from build123d import *

# Parameters (mm, degrees)
SKETCH1_W           = 60.00000000000001
SKETCH1_H           = 32
BOSS_EXTRUDE1_DEPTH = 5.3
BOSS_EXTRUDE2_DEPTH = 60
SKETCH4_R           = 5.050000000000001
BOSS_EXTRUDE3_DEPTH = 5
BOSS_EXTRUDE4_DEPTH = 15
BOSS_EXTRUDE5_DEPTH = 5.3
CUT_EXTRUDE1_DEPTH  = 10
CUT_EXTRUDE2_DEPTH  = 5
CUT_EXTRUDE3_DEPTH  = 5
CUT_EXTRUDE4_START  = -15
SKETCH4_4_R         = 5.050000000000001
CUT_EXTRUDE4_DEPTH  = 15
FILLET1_R           = 1


with BuildPart() as part:
    # Sketch1 → Boss-Extrude1 (new body)
    with BuildSketch(Plane.XY):
        with Locations((30.000000000000004, 16)):
            Rectangle(SKETCH1_W, SKETCH1_H)
    extrude(amount=BOSS_EXTRUDE1_DEPTH)

    # Sketch3 → Boss-Extrude2 (add)
    with BuildSketch(Plane.ZY):
        Polygon((5.29999999999999, 32), (5.29999999999999, 32.5), (0, 32), align=None)
        Polygon((5.3, -0.5), (5.3, 0), (0, 0), align=None)
    extrude(amount=-BOSS_EXTRUDE2_DEPTH)

    # Sketch4 → Boss-Extrude3 (add)
    # profile 1 of 9: a face of its own
    with BuildSketch(Plane.XY.offset(5.3)):
        Polygon((1.3289678218773275, 32.5), (24.983548935155518, 32.5), (1.5086509412101563, 34.55378745189766), align=None)
    # profile 2 of 9: a face of its own
    with BuildSketch(Plane.XY.offset(5.3)):
        Polygon((0, 2.5635425050841554), (35.01645106484395, -0.4999999999999578), (58.671032178122694, -0.5000000000000004), (59.999999999999964, 14.690171712744215), (60, 29.43645749491585), (24.983548935155518, 32.5), (1.3289678218773275, 32.5), (-4e-15, 17.309828287255154), align=None)
        with Locations((30, 16)):
            Circle(SKETCH4_R, mode=Mode.SUBTRACT)
    # profile 3 of 9: a face of its own
    with BuildSketch(Plane.XY.offset(5.3)):
        Polygon((0, -0.5000000000000004), (35.01645106484395, -0.5000000000000004), (0, 2.5635425050841554), align=None)
    # profile 4 of 9: a face of its own
    with BuildSketch(Plane.XY.offset(5.3)):
        Polygon((58.055570345051585, -7.534760942356384), (58.49134905878986, -2.553787451897688), (35.01645106484395, -0.4999999999999578), (0, -0.5000000000000004), (0, 2.5635425050841576), (-1.2803328267148615, 2.675557112961807), (-1.7161115404531533, -2.3054163774969894), align=None)
    # profile 5 of 9: a face of its own
    with BuildSketch(Plane.XY.offset(5.3)):
        Polygon((35.01645106484395, -0.4999999999999578), (58.49134905878986, -2.5537874518976778), (58.671032178122694, -0.5000000000000071), align=None)
    # profile 6 of 9: a face of its own
    with BuildSketch(Plane.XY.offset(5.3)):
        Polygon((59.999999999999964, 14.690171712744215), (61.28033282671488, 29.324442887038195), (60, 29.436457494915846), align=None)
    # profile 7 of 9: a face of its own
    with BuildSketch(Plane.XY.offset(5.3)):
        Polygon((24.983548935155518, 32.5), (60, 29.436457494915846), (60, 32.5), align=None)
    # profile 8 of 9: a face of its own
    with BuildSketch(Plane.XY.offset(5.3)):
        Polygon((60, 29.436457494915846), (61.28033282671488, 29.324442887038195), (61.71611154045317, 34.305416377497), (1.944429654948438, 39.5347609423564), (1.5086509412101552, 34.55378745189767), (24.983548935155518, 32.5), (60, 32.5), align=None)
    # profile 9 of 9: a face of its own
    with BuildSketch(Plane.XY.offset(5.3)):
        Polygon((-1.2803328267148615, 2.675557112961807), (0, 2.5635425050841554), (0, 17.309828287255158), align=None)
    extrude(amount=BOSS_EXTRUDE3_DEPTH)

    # Sketch4<3> → Boss-Extrude4 (add)
    with BuildSketch(Plane.XY.offset(5.3)):
        Polygon((60, 29.436457494915846), (61.28033282671488, 29.324442887038195), (61.71611154045317, 34.305416377497), (1.944429654948438, 39.5347609423564), (1.5086509412101552, 34.55378745189767), (24.983548935155518, 32.5), (60, 32.5), align=None)
        Polygon((24.983548935155518, 32.5), (60, 29.436457494915846), (60, 32.5), align=None)
        Polygon((58.055570345051585, -7.534760942356384), (58.49134905878986, -2.553787451897688), (35.01645106484395, -0.4999999999999578), (0, -0.5000000000000004), (0, 2.5635425050841576), (-1.2803328267148615, 2.675557112961807), (-1.7161115404531533, -2.3054163774969894), align=None)
        Polygon((0, -0.5000000000000004), (35.01645106484395, -0.5000000000000004), (0, 2.5635425050841554), align=None)
    extrude(amount=BOSS_EXTRUDE4_DEPTH)

    # Sketch6 → Boss-Extrude5 (add)
    with BuildSketch(Plane(origin=(0, 0, 5.3), x_dir=(-1, 0, 0), z_dir=(0, 0, -1))):
        Polygon((-2.2e-16, 17.3098282872552), (0, -0.5000000000000004), (1.558158074478129, -0.499999999999997), align=None)
        Polygon((-60.00000000000001, 14.690171712744698), (-60, 32.5), (-61.55815807447815, 32.5), align=None)
    extrude(amount=BOSS_EXTRUDE5_DEPTH)

    # Sketch5 → Cut-Extrude1 (cut)
    with BuildSketch(Plane.XY.offset(5.3)):
        Polygon((58.671032178122694, -0.5000000000000004), (60, -0.5000000000000004), (60.00000000000001, 14.690171712744698), align=None)
        Polygon((1.328967821877318, 32.5), (0, 32.5), (2.2e-16, 17.3098282872552), align=None)
    extrude(amount=-CUT_EXTRUDE1_DEPTH, mode=Mode.SUBTRACT)

    # Sketch7 → Cut-Extrude2 (cut)
    with BuildSketch(Plane(origin=(0, 0, 0), x_dir=(0, 0, -1), z_dir=(1, -1e-17, 0))):
        Polygon((0, -0.5000000000000004), (3.2e-16, 3.5e-15), (-5.3, -0.5000000000000004), align=None)
    extrude(amount=-CUT_EXTRUDE2_DEPTH, mode=Mode.SUBTRACT)

    # Sketch8 → Cut-Extrude3 (cut)
    with BuildSketch(Plane.ZY.offset(-60.000000000000014)):
        Polygon((5.299999999999987, 32.49999999999998), (0, 31.99999999999998), (0, 32.49999999999998), align=None)
    extrude(amount=-CUT_EXTRUDE3_DEPTH, mode=Mode.SUBTRACT)

    # Sketch4<4> → Cut-Extrude4 (cut)
    with BuildSketch(Plane.XY.offset(5.3).offset(CUT_EXTRUDE4_START)):
        with Locations(Location((30, 16, 0), (0, 0, 180))):
            Circle(SKETCH4_4_R)
    extrude(amount=CUT_EXTRUDE4_DEPTH, mode=Mode.SUBTRACT)

    # Fillet1
    fillet1_edges = [part.edges().sort_by_distance(p)[0] for p in [
        (-1.637134807465641, -1.402708188748493, 5.3),
        (58.692904344004184, -0.25000000000000244, 2.65),
        (1.307095655995838, 32.25, 2.6499999999999977),
        (-0.11459512630040658, 16.000000000000004, 0),
        (-1.5362859085966487, -0.24999999999999853, 2.65),
        (60.11459512630042, 15.999999999999996, 0),
        (61.53628590859667, 32.25, 2.6499999999999937),
        (35.05, 16, 0),
        (58.36330126158714, -4.017380471178193, 5.3),
        (61.63713480746566, 33.4027081887485, 5.3),
        (31.830270597700803, 36.920088659926705, 5.3),
        (1.6366987384128773, 36.0173804711782, 5.299999999999997),
        (1.944429654948438, 39.5347609423564, 12.8),
        (28.169729402299218, -4.920088659926687, 5.3),
        (-1.7161115404531533, -2.3054163774969894, 12.8),
        (58.055570345051585, -7.534760942356385, 12.8),
        (61.71611154045317, 34.305416377497, 12.8),
        (24.95, 16, 10.3),
        (31.399818616414773, 32, 0),
        (28.60018138358524, 1.74e-15, -8e-17),
        (0.11415905724764364, 18.61467228242972, 10.3),
        (59.885840942752374, 13.38532771757026, 10.3),
        (31.394491883962516, 31.939115169467932, 10.3),
        (1.7265402980792965, 37.04427419712704, 20.3),
        (1.5086509412101559, 34.55378745189766, 15.3),
        (31.39449188396252, 31.93911516946793, 20.3),
        (61.28033282671488, 29.324442887038195, 15.3),
        (31.830270597700803, 36.920088659926705, 20.3),
        (61.498222183584026, 31.814929632267596, 20.3),
        (28.605508116037498, 0.06088483053206062, 10.3),
        (58.49134905878986, -2.5537874518976826, 15.3),
        (-1.2803328267148655, 2.675557112961773, 15.3),
        (58.27345970192072, -5.044274197127036, 20.3),
        (28.605508116037498, 0.06088483053204508, 20.3),
        (-1.4982221835840113, 0.18507036773237484, 20.3),
        (28.169729402299218, -4.920088659926687, 20.3),
    ]]
    fillet(fillet1_edges, radius=FILLET1_R)


solid = part.part
For this review, take the finished solid that the model builds, in its own axes (mm). A direction names the side the tool comes from. Give positions to 0.01 mm unless a question says otherwise; leave off trailing zeros. Loops run counter-clockwise (first coordinate to the right, second up) from the corner with the lowest first, then second, coordinate; pieces in that order, holes last.
Item 1: Insertion check: pin 1 (12 mm diameter, centred on x = 41, z = 11.5, fed in from +Y); pin 2 (1 mm diameter, centred on x = 38, z = 3.5, fed in from -Y); pin 3 (5 mm diameter, centred on x = 11.5, z = 18, fed in from +Y); pin 4 (6 mm diameter, centred on x = 30, y = 16, fed in from +Z). Each pin has a flat end and moves straight along its axis. Give the tip position at first contact, or say it passes through.
Item 2: Take a section at B-B, the plane z = 8.25. State the section outline as (x, y) points.
Item 3: Take a section at A-A, the plane z = 13. State the section outline as (x, y) points, and give its area (3 significant figures).
Item 4: Tool access review of faces 1 (the flat face through (28, -2, 20.3)), 2 (the flat face through (35, -3, 5.3)), 3 (the flat face through (29.01, 0.025, 15.244)), 4 (the flat face through (30.99, 31.975, 15.244)): name each direction out of +Z, -Z, +X, -X, +Y, -Y from which nothing blocks a thin tool from reaching the whole face with its end or side.
Item 5: Draft analysis for pull direction Y (two halves, no side actions). For faces 5 (the flat face through (25, 35, 5.3)), 6 (the cylindrical face through (30.964, 31.675, 10.585)), 7 (the flat face through (59.91, 13.66, 8.24)), 8 (the cylindrical face through (31.4, 36.67, 5.6)), state which applies: +Y half, -Y half, draft (parallel to the pull), parting line (faces both ways), or undercut.
Item 6: For line 1 along Z through (x, y) = (25, 24.5); line 2 along Y through (x, z) = (30, 6.1); line 3 along X through (y, z) = (16, 7.8), list the stretches that pass through material, from the lowest coordinate up.
Calculated:
1. pin 1: stops at y = 36.64
1. pin 2: stops at y = -0.38
1. pin 3: stops at y = 38.92
1. pin 4: passes through
2. outline: (-1.63, -1.31) arc R1 ccw to (-0.72, -2.39) - (57.06, -7.45) arc R1 ccw to (58.14, -6.54) - (61.63, 33.31) arc R1 ccw to (60.72, 34.39) - (2.94, 39.45) arc R1 ccw to (1.86, 38.54) - close; hole circle Ø10.1 at (30, 16)
3. outline: (-1.63, -1.31) arc R1 ccw to (-0.72, -2.39) - (57.06, -7.45) arc R1 ccw to (58.14, -6.54) - (58.4, -3.55) arc R1 ccw to (57.5, -2.47) - (-0.28, 2.59) arc R1 ccw to (-1.37, 1.68) - close; (1.6, 35.55) arc R1 ccw to (2.5, 34.47) - (60.28, 29.41) arc R1 ccw to (61.37, 30.32) - (61.63, 33.31) arc R1 ccw to (60.72, 34.39) - (2.94, 39.45) arc R1 ccw to (1.86, 38.54) - close
3. area: 598 mm2
4. face 1: +Z, +X, -X, +Y, -Y
4. face 2: -Z, +X, -X, -Y
4. face 3: +Z, +X
4. face 4: +Z, -X
5. face 5: draft
5. face 6: undercut
5. face 7: -Y half
5. face 8: +Y half
6. line 1: z = 0 to 10.3
6. line 2: y = -5.06 to 10.95, 21.05 to 37.06
6. line 3: x = -0.11 to 24.95, 35.05 to 60.11
